```python
from build123d import *

# Parameters (mm, degrees)
SKETCH2_R           = 30
BOSS_EXTRUDE1_DEPTH = 4
SKETCH3_R           = 12
BOSS_EXTRUDE2_DEPTH = 25
SKETCH4_R           = 9.5
CUT_EXTRUDE1_DEPTH  = 25
SKETCH5_R           = 8
CUT_EXTRUDE2_DEPTH  = 20
SKETCH6_R           = 1.5
CUT_EXTRUDE10_DEPTH = 4
SKETCH8_R           = 2
CUT_EXTRUDE14_DEPTH = 25


with BuildPart() as part:
    # Sketch2 → Boss-Extrude1 (new body)
    with BuildSketch(Plane.XY):
        Circle(SKETCH2_R)
    extrude(amount=BOSS_EXTRUDE1_DEPTH)

    # Sketch3 → Boss-Extrude2 (add)
    with BuildSketch(Plane.XY.offset(4)):
        Circle(SKETCH3_R)
    extrude(amount=BOSS_EXTRUDE2_DEPTH)

    # Sketch4 → Cut-Extrude1 (cut)
    with BuildSketch(Plane(origin=(0, 0, 0), x_dir=(-1, 0, 0), z_dir=(0, 0, -1))):
        Circle(SKETCH4_R)
    extrude(amount=-CUT_EXTRUDE1_DEPTH, mode=Mode.SUBTRACT)

    # Sketch5 → Cut-Extrude2 (cut)
    with BuildSketch(Plane(origin=(0, 0, 25), x_dir=(-1, 0, 0), z_dir=(0, 0, -1))):
        Circle(SKETCH5_R)
    extrude(amount=-CUT_EXTRUDE2_DEPTH, mode=Mode.SUBTRACT)

    # Sketch6 → Cut-Extrude10 (cut)
    with BuildSketch(Plane(origin=(0, 0, 0), x_dir=(-1, 0, 0), z_dir=(0, 0, -1))):
        with Locations((0, 13)):
            Circle(SKETCH6_R)
        with Locations((13, 0)):
            Circle(SKETCH6_R)
        with Locations((0, -13)):
            Circle(SKETCH6_R)
        with Locations((-13, 0)):
            Circle(SKETCH6_R)
    extrude(amount=-CUT_EXTRUDE10_DEPTH, mode=Mode.SUBTRACT)

    # Sketch8 → Cut-Extrude14 (cut)
    with BuildSketch(Plane.XY.offset(29)):
        with Locations((0.039889562, 13)):
            Circle(SKETCH8_R)
        with Locations((0, -13)):
            Circle(SKETCH8_R)
        with Locations((13, 0)):
            Circle(SKETCH8_R)
        with Locations((-13, 0)):
            Circle(SKETCH8_R)
    extrude(amount=-CUT_EXTRUDE14_DEPTH, mode=Mode.SUBTRACT)


solid = part.part
```
Verification items for the finished model (mm, model axes). A direction names the side the tool comes from. Give positions to 0.01 mm unless a question says otherwise; leave off trailing zeros. Loops run counter-clockwise (first coordinate to the right, second up) from the corner with the lowest first, then second, coordinate; pieces in that order, holes last. Notation, with made-up numbers: M -6,86 L 40,86 A16 cw 40,98 Z; hole C 42,56.5 d4. An arc over 180 degrees is marked long. One line per question, with ' | ' between items.
Item 1: Section check A-A, the plane y = 0. Record the cut outline in (x, z), plus the area to 3 significant figures.
Completed:
outline: M -30,0 L -14.5,0 L -14.5,4 L -30,4 Z; M -11.5,0 L -9.5,0 L -9.5,25 L -8,25 L -8,29 L -11,29 L -11,4 L -11.5,4 Z; M 8,25 L 9.5,25 L 9.5,0 L 11.5,0 L 11.5,4 L 11,4 L 11,29 L 8,29 Z; M 14.5,0 L 30,0 L 30,4 L 14.5,4 Z | area: 227 mm^2
Item 2: Depth check by flat-ended pin: P1, Ø10, axis at x = -12.5, z = 18.5, coming from the -Y side; P2, Ø18.5, axis at x = 0, y = 0, coming from the -Z side; P3, Ø1, axis at y = 7.5, z = 13.5, coming from the +X side. Enter the tip coordinate at first touch or a pass-through.
Completed:
P1: stops at y = -9.37 | P2: stops at z = 25 | P3: stops at x = 9.75
Item 3: Thickness scan on line 1 (Y direction, x = 0, z = 3); line 2 (Y direction, x = 0, z = 14.75); line 3 (Y direction, x = 0, z = 27.55). Record the ranges inside material, lowest first. Write a range as [from, to].
Completed:
line 1: y = [-30, -14.5], [-11.5, -9.5], [9.5, 11.5], [14.5, 30] | line 2: y = [-11, -9.5], [9.5, 11] | line 3: y = [-11, -8], [8, 11]
Item 4: Draft check along X on faces 1 (the face through (-8.395, 8.575, 16.325)), 2 (the face through (14.5, 0.07, 1.97)), 3 (the face through (11, 0, 17)). Enter one of: +X half, -X half, draft (parallel to the pull), parting line (faces both ways), or undercut.
Completed:
face 1: -X half | face 2: undercut | face 3: +X half
Item 5: Tool access check on faces 4 (the face through (-8.56, -8.41, 16.32)), 5 (the face through (8.41, -8.56, 16.32)), 6 (the face through (0, 11, 17)), 7 (the face through (4.3, -7, 25)). Record the directions out of +Z, -Z, +X, -X, +Y, -Y that give a thin tool (end or side, any length) a straight path to the whole face; none if there is none.
Completed:
face 4: +Z, -X, -Y | face 5: +Z, +X, -Y | face 6: +Z, +Y | face 7: -Z
Item 6: Section check C-C, the plane x = 6. Record the cut outline in (y, z).
Completed:
outline: M -29.39,0 L -7.37,0 L -7.37,25 L -5.29,25 L -5.29,29 L -10.39,29 L -10.39,4 L -29.39,4 Z; M 5.29,25 L 7.37,25 L 7.37,0 L 29.39,0 L 29.39,4 L 10.39,4 L 10.39,29 L 5.29,29 Z
Item 7: Section check B-B, the plane z = 7. Record the cut outline in (x, y).
Completed:
outline: M -11.88,-1.66 A12 ccw -1.66,-11.88 A2 cw 1.66,-11.88 A12 ccw 11.88,-1.66 A2 cw 11.88,1.66 A12 ccw 1.7,11.88 A2 cw -1.62,11.89 A12 ccw -11.88,1.66 A2 cw Z; hole C 0,0 d19
Item 8: Section check D-D, the plane y = -13. Record the cut outline in (x, z).
Completed:
outline: M -27.04,0 L -1.5,0 L -1.5,4 L -27.04,4 Z; M 1.5,0 L 27.04,0 L 27.04,4 L 1.5,4 Z
